For this review, take the finished solid that the model builds, in its own axes (mm). A direction names the side the tool comes from. Give positions to 0.01 mm unless a question says otherwise; leave off trailing zeros. Loops run counter-clockwise (first coordinate to the right, second up) from the corner with the lowest first, then second, coordinate; pieces in that order, holes last. Notation, with made-up numbers: M 15,-1.75 L 58,-1.75 A35 ccw 58,33.25 Z; hole C -18.75,44.25 d9. An arc over 180 degrees is marked long. Use CSV: the item, a comma, the result in double quotes. Start each with the question number.
1. The part is to be moulded in two halves that separate along X. For faces 6 (the face through (-6, 6.25, -5)), 7 (the face through (6.45, 0, -5)), 8 (the face through (-2.3, -5.2, -7.6)), say which applies: pulls with the +X half, pulls with the -X half, needs draft (parallel to the pull), parting line crosses it, or undercut.
2. Take a section at D-D, the plane z = -3.5. Write out the cut boundary in (x, y).
3. Insertion check: P1, Ø3, axis at x = 2, y = -3.5, coming from the -Z side; P2, Ø1, axis at x = 5, y = 4.5, coming from the -Z side; P3, Ø0.8, axis at x = -3.5, z = -9.5, coming from the -Y side. Each pin has a flat end and moves straight along its axis. Give the tip position at first contact, or say it passes through.
4. Tool access review of faces 1 (the face through (0, 5.95, -5)), 2 (the face through (2.3, -2, -10.5)), 3 (the face through (0, -1, -9.55)), 4 (the face through (0, -5.95, -5)), 5 (the face through (2.3, 5.2, -7.6)): name each direction out of +Z, -Z, +X, -X, +Y, -Y from which nothing blocks a thin tool from reaching the whole face with its end or side.
5. Take a section at C-C, the plane z = -7.25. Write out the cut boundary in (x, y).
6. Take a section at A-A, the plane x = -4.5. Write out the cut boundary in (y, z), and give its area (3 significant figures).
7. To check wall thickness, follow line 1 (Y direction, x = -2, z = -1.5); line 2 (X direction, y = -5.5, z = -6.75). State the ranges of each line that lie inside material, in increasing order. Write a range as [from, to].
8. Take a section at B-B, the plane y = 2.5. Write out the cut boundary in (x, z), and give its area (3 significant figures).
from build123d import *

# Parameters (mm, degrees)
SKETCH_W        = 12.9
SKETCH_H        = 12.5
PAD_DEPTH       = 9.25
FILLET_R        = 0.25
SKETCH001_W     = 9.8
SKETCH001_H     = 0.3
POCKET_DEPTH    = 9.251
SKETCH002_R     = 0.75
POCKET001_DEPTH = 4
PAD001_DEPTH    = 3.95
FILLET001_R     = 0.44
PAD002_DEPTH    = 5.4
FILLET002_R     = 0.44


with BuildPart() as part:
    # Sketch → Pad (new body)
    with BuildSketch(Plane.XY):
        Rectangle(SKETCH_W, SKETCH_H)
    extrude(amount=-PAD_DEPTH)

    # Fillet
    fillet_edges = [part.edges().sort_by_distance(p)[0] for p in [
        (6.45, -6.25, -4.625),
        (-6.45, -6.25, -4.625),
        (-6.45, 6.25, -4.625),
        (6.45, 6.25, -4.625),
    ]]
    fillet(fillet_edges, radius=FILLET_R)

    # Sketch001 (on Face2 of Fillet) → Pocket (cut, through all)
    with BuildSketch(Plane.XY):
        with Locations((0, -6.1)):
            Rectangle(SKETCH001_W, SKETCH001_H)
        with Locations((0, 6.1)):
            Rectangle(SKETCH001_W, SKETCH001_H)
    extrude(amount=-POCKET_DEPTH, mode=Mode.SUBTRACT)

    # Sketch002 (on Face4 of Pocket) → Pocket001 (cut)
    with BuildSketch(Plane(origin=(0, 0, -9.25), x_dir=(1, 0, 0), z_dir=(0, 0, -1))):
        with Locations((-2.3, 5.95)):
            Circle(SKETCH002_R)
        with Locations((2.3, 5.95)):
            Circle(SKETCH002_R)
        with Locations((-2.3, -5.95)):
            Circle(SKETCH002_R)
        with Locations((2.3, -5.95)):
            Circle(SKETCH002_R)
    extrude(amount=-POCKET001_DEPTH, mode=Mode.SUBTRACT)

    # Sketch003 → Pad001 (join, symmetric)
    with BuildSketch(Plane.XZ):
        with BuildLine():
            ThreePointArc((-1.85, -9.25), (-2.3, -8.8), (-2.75, -9.25))
            Line((-2.75, -9.25), (-2.75, -9.75))
            ThreePointArc((-2.75, -9.75), (-2.3, -10.2), (-1.85, -9.75))
            Line((-1.85, -9.75), (-1.85, -9.25))
        make_face()
        with BuildLine():
            ThreePointArc((2.75, -9.25), (2.3, -8.8), (1.85, -9.25))
            Line((1.85, -9.25), (1.85, -9.75))
            ThreePointArc((1.85, -9.75), (2.3, -10.2), (2.75, -9.75))
            Line((2.75, -9.75), (2.75, -9.25))
        make_face()
    extrude(amount=PAD001_DEPTH, both=True)

    # Fillet001
    fillet001_edges = [part.edges().sort_by_distance(p)[0] for p in [
        (-2.3, 3.95, -10.2),
        (2.3, 3.95, -10.2),
        (2.3, -3.95, -10.2),
        (-2.3, -3.95, -10.2),
    ]]
    fillet(fillet001_edges, radius=FILLET001_R)

    # Sketch004 → Pad002 (join, symmetric)
    with BuildSketch(Plane.YZ):
        with BuildLine():
            ThreePointArc((0.45, -9.25), (0, -8.8), (-0.45, -9.25))
            Line((-0.45, -9.25), (-0.45, -10))
            ThreePointArc((-0.45, -10), (0, -10.45), (0.45, -10))
            Line((0.45, -10), (0.45, -9.25))
        make_face()
    extrude(amount=PAD002_DEPTH, both=True)

    # Fillet002
    fillet002_edges = [part.edges().sort_by_distance(p)[0] for p in [
        (-5.4, 0, -10.45),
        (5.4, 0, -10.45),
    ]]
    fillet(fillet002_edges, radius=FILLET002_R)


with BuildPart() as part_1:
    # Body placement: moved
    add(part.part.moved(Location((0, 0, -0.3))))


solid = part_1.part
Result set:
1,face 6,"needs draft"
1,face 7,"pulls with the +X half"
1,face 8,"undercut"
2,outline,"M -6.45,-6 A0.25 ccw -6.2,-6.25 L -4.9,-6.25 L -4.9,-5.95 L 4.9,-5.95 L 4.9,-6.25 L 6.2,-6.25 A0.25 ccw 6.45,-6 L 6.45,6 A0.25 ccw 6.2,6.25 L 4.9,6.25 L 4.9,5.95 L -4.9,5.95 L -4.9,6.25 L -6.2,6.25 A0.25 ccw -6.45,6 Z"
3,P1,"z = -10.5"
3,P2,"z = -9.55"
3,P3,"y = -5.95"
4,face 1,"+Z, -Z, +Y"
4,face 2,"-Z, -Y"
4,face 3,"-Z"
4,face 4,"+Z, -Z, -Y"
4,face 5,"-Z, +Y"
5,outline,"M -6.45,-6 A0.25 ccw -6.2,-6.25 L -4.9,-6.25 L -4.9,-5.95 L -3.05,-5.95 A0.75 cw -1.55,-5.95 L 1.55,-5.95 A0.75 cw 3.05,-5.95 L 4.9,-5.95 L 4.9,-6.25 L 6.2,-6.25 A0.25 ccw 6.45,-6 L 6.45,6 A0.25 ccw 6.2,6.25 L 4.9,6.25 L 4.9,5.95 L 3.05,5.95 A0.75 cw 1.55,5.95 L -1.55,5.95 A0.75 cw -3.05,5.95 L -4.9,5.95 L -4.9,6.25 L -6.2,6.25 A0.25 ccw -6.45,6 Z"
6,outline,"M -5.95,-9.55 L -0.45,-9.55 L -0.45,-10.3 A0.45 ccw 0.45,-10.3 L 0.45,-9.55 L 5.95,-9.55 L 5.95,-0.3 L -5.95,-0.3 Z"
6,area,"111 mm2"
7,line 1,"[-5.95, 5.95]"
7,line 2,"[-6.45, -2.9], [-1.7, 1.7], [2.9, 6.45]"
8,outline,"M -6.45,-9.55 L -2.75,-9.55 L -2.75,-10.05 A0.45 ccw -1.85,-10.05 L -1.85,-9.55 L 1.85,-9.55 L 1.85,-10.05 A0.45 ccw 2.75,-10.05 L 2.75,-9.55 L 6.45,-9.55 L 6.45,-0.3 L -6.45,-0.3 Z"
8,area,"121 mm2"
